Could you check a few things on this model? Use its own coordinates, in mm. A direction names the side the tool comes from. Give positions to 0.01 mm unless a question says otherwise; leave off trailing zeros. Loops run counter-clockwise (first coordinate to the right, second up) from the corner with the lowest first, then second, coordinate; pieces in that order, holes last. Notation, with made-up numbers: M 35.5,88 L 41.5,88 A32 ccw 41.5,123 Z; hole C 5.5,-37 d4. An arc over 180 degrees is marked long. Return JSON: item names as keys, results as strings. Group by question number.
1. Please list where these lines run through material, in increasing order: line 1 (Z direction, x = 0, y = 11.5); line 2 (X direction, y = 13.5, z = -8.5); line 3 (X direction, y = 10, z = 0).
2. For faces 1 (the flat face through (2.608, 7.888, 24.465)), 2 (the flat face through (14.632, 11.014, 10.4)), 3 (the flat face through (15.81, 7.89, 4.42)), which set-ups out of +Z, -Z, +X, -X, +Y, -Y let a thin tool reach every point of the face, with its end or its side?
3. If we section it at D-D (x = 0): Write out the boundary of the cut face in (y, z), plus the area to 3 significant figures.
4. If we mould it in two halves opening along X, with no side actions, what happens to faces 4 (the flat face through (21.43, 4.33, 12.68)), 5 (the cylindrical face through (-4.37, 7.89, 20.2)), 6 (the flat face through (16.497, 6.15, 11.227))? For each: +X half, -X half, draft (parallel to the pull), parting line (faces both ways), or undercut.
5. If we section it at C-C (x = -15): Write out the boundary of the cut face in (y, z).
6. If we section it at A-A (z = 15.8): Write out the boundary of the cut face in (x, y).
7. If we section it at B-B (y = 7.25): State how many separate pieces and enclosed holes the cut face has, plus the area to 3 significant figures.
8. For pin 1 (6 mm diameter, centred on y = 5.5, z = -7.5, fed in from -X); pin 2 (6 mm diameter, centred on x = 17.5, y = 8, fed in from -Z); pin 3 (4 mm diameter, centred on x = 22.5, y = 2.5, fed in from -Z), each with a flat end and sliding along its axis, tell me the tip position at first contact or that it passes through.
Solid Edge part; units mm, degrees
sketch "Sketch1" plane through (0, 0, 0) normal (0, -1, 0) x (1, 0, 0)
  line L0 (-5.3694, 18.9) -> (-19.0694, -4.8291)
  arc A0 (-13.7, -14.1291) -> (-19.0694, -4.8291) centre (-13.7, -7.9291) cw
  line L1 (-13.7, -14.1291) -> (13.7, -14.1291)
  arc A1 (19.0694, -4.8291) -> (13.7, -14.1291) centre (13.7, -7.9291) cw
  line L2 (5.3694, 18.9) -> (19.0694, -4.8291)
  arc A2 (-5.3694, 18.9) -> (5.3694, 18.9) centre (0, 15.8) cw
  dimension "D1" = 5.3694
extrude "Protrusion1" add sketch "Sketch1" against normal blind 16
sketch "Sketch2" plane through (0, 0, 0) normal (0, -1, 0) x (1, 0, 0)
  circle A0 centre (-13.7, -7.9291) radius 2.2
  circle A1 centre (13.7, -7.9291) radius 2.2
  circle A2 centre (0, 15.8) radius 2.2
extrude "Cutout1" cut sketch "Sketch2" against normal blind 457.8755
sketch "Sketch3" plane through (0, 0, 0) normal (0, -1, 0) x (1, 0, 0)
  circle A0 centre (0, 0) radius 6
extrude "Cutout2" cut sketch "Sketch3" against normal blind 434.4917
sketch "Sketch4" plane through (0, 0, 3.9355) normal (0, -1, 0) x (-0.5, 0, 0.866)
  line L0 (-23.325, -5.9323) -> (-23.325, -18.9323)
  line L1 (-23.325, -18.9323) -> (16.475, -18.9323)
  line L2 (16.475, -18.9323) -> (16.475, -5.9323)
  line L3 (12.7755, -8.7037) -> (16.475, -5.9323)
  line L4 (-20.9306, -8.7037) -> (12.7755, -8.7037)
  line L5 (-20.9306, -5.9323) -> (-20.9306, -8.7037)
  line L6 (-23.325, -5.9323) -> (-20.9306, -5.9323)
  dimension "D1" = 23.325
extrude "Protrusion2" add sketch "Sketch4" against normal up to vertex (16 mm away)
sketch "Sketch5" plane through (3.1086, 0, 6.2098) normal (0, -1, 0) x (-0.5, 0, 0.866)
  line L0 (-8.3403, 2.4623) -> (-8.3403, -10.1029)
  line L1 (-8.3403, -10.1029) -> (0.6597, -10.1029)
  line L2 (0.6597, -10.1029) -> (0.6597, 2.4623)
  line L3 (0.6597, 2.4623) -> (-8.3403, 2.4623)
extrude "ExtrudedCutout_18" cut sketch "Sketch5" against normal blind 196.9446
sketch "Sketch6" plane through (13.7782, 8, 7.9355) normal (-0.866, 0, -0.5) x (0, -1, 0)
  line L0 (-2, 3.4641) -> (2, 3.4641)
  line L1 (-4, 0) -> (-2, 3.4641)
  line L2 (-2, -3.4641) -> (-4, 0)
  line L3 (2, -3.4641) -> (-2, -3.4641)
  line L4 (5.4641, 0) -> (2, -3.4641)
  line L5 (2, 3.4641) -> (5.4641, 0)
extrude "ExtrudedCutout_19" cut sketch "Sketch6" against normal blind 4
sketch "Sketch7" plane through (18.1083, 8, 10.4355) normal (0.866, 0, 0.5) x (-0.5, 0, 0.866)
  line L0 (-19.9, 8) -> (19.9, 8)
  line L1 (19.9, -8) -> (19.9, 8)
  line L2 (-19.9, -8) -> (19.9, -8)
  line L3 (-19.9, -8) -> (-19.9, 8)
extrude "ExtrudedProtrusion_14" add sketch "Sketch7" along normal blind 4
sketch "Sketch8" plane through (21.5724, 8, 12.4355) normal (0.866, 0, 0.5) x (-0.5, 0, 0.866)
  line L0 (-1.5556, 1.5556) -> (0, 3.1113)
  line L1 (0, 3.1113) -> (1.5556, 1.5556)
  arc A0 (1.5556, 1.5556) -> (-1.5556, 1.5556) centre (0, 0) cw
extrude "ExtrudedCutout_20" cut sketch "Sketch8" against normal blind 25.1595
Answer:
{
 "1": {"line 1": "z = -14.13 to -6, 6 to 13.6, 18 to 22.96", "line 2": "x = -19.87 to -15.82, -11.58 to 11.58, 15.82 to 25.11", "line 3": "x = -16.28 to -6, 9.03 to 28.75"},
 "2": {"face 1": "+Z, -X, +Y, -Y", "face 2": "none", "face 3": "+Y, -Y"},
 "3": {"outline": "M 0,-14.13 L 16,-14.13 L 16,-6 L 0,-6 Z; M 0,6 L 16,6 L 16,13.6 L 0,13.6 Z; M 0,18 L 16,18 L 16,22.96 L 0,22.96 Z", "area": "331 mm²"},
 "4": {"face 4": "+X half", "face 5": "-X half", "face 6": "undercut"},
 "5": {"outline": "M 0,-13.99 L 16,-13.99 L 16,-9.7 L 0,-9.7 Z; M 0,-6.15 L 16,-6.15 L 16,2.22 L 0,2.22 Z"},
 "6": {"outline": "M -7.16,0 L -2.2,0 L -2.2,16 L -7.16,16 Z; M 2.2,0 L 19.63,0 L 19.63,16 L 2.2,16 Z"},
 "7": {"separate pieces": "1", "enclosed holes": "3", "area": "1,100 mm²"},
 "8": {"pin 1": "stops at x = -19.9", "pin 2": "stops at z = -14.08", "pin 3": "stops at z = -11.16"}
}
